```python
from build123d import *

# Parameters (mm, degrees)
SKETCH1_W           = 144
SKETCH1_H           = 71.25
BOSS_EXTRUDE1_DEPTH = 1
SKETCH2_W           = 13.75
SKETCH2_H           = 13.75
CUT_EXTRUDE1_DEPTH  = 81.33766629
SKETCH3_W           = 13.75
SKETCH3_H           = 13.75
CUT_EXTRUDE2_DEPTH  = 81.33766629
SKETCH4_W           = 7.5
SKETCH4_H           = 7.5
CUT_EXTRUDE6_DEPTH  = 81.33766629


with BuildPart() as part:
    # Sketch1 → Boss-Extrude1 (new body)
    with BuildSketch(Plane(origin=(0, 0, 0), x_dir=(1, 0, 0), z_dir=(0, 1, 0))):
        Rectangle(SKETCH1_W, SKETCH1_H)
    extrude(amount=BOSS_EXTRUDE1_DEPTH)

    # Sketch2 → Cut-Extrude1 (cut, through all)
    with BuildSketch(Plane(origin=(0, 1, 0), x_dir=(1, 0, 0), z_dir=(0, 1, 0))):
        with Locations((-36.375, 18.75)):
            Rectangle(SKETCH2_W, SKETCH2_H)
        with Locations((-55.125, 0)):
            Rectangle(SKETCH2_W, SKETCH2_H)
        with Locations((-36.375, -18.75)):
            Rectangle(SKETCH2_W, SKETCH2_H)
        with Locations((-17.625, 0)):
            Rectangle(SKETCH2_W, SKETCH2_H)
    cut_extrude1 = extrude(amount=-CUT_EXTRUDE1_DEPTH, mode=Mode.SUBTRACT)

    # Mirror1: Cut-Extrude1 across plane
    add(cut_extrude1.mirror(Plane(origin=(0, 0, 0), x_dir=(0, 0, 1), z_dir=(1, 0, 0))), mode=Mode.SUBTRACT)

    # Sketch3 → Cut-Extrude2 (cut, through all)
    with BuildSketch(Plane(origin=(0, 1, 0), x_dir=(1, 0, 0), z_dir=(0, 1, 0))):
        with Locations((0, 18.75)):
            Rectangle(SKETCH3_W, SKETCH3_H)
    extrude(amount=-CUT_EXTRUDE2_DEPTH, mode=Mode.SUBTRACT)

    # Sketch4 → Cut-Extrude6 (cut, through all)
    with BuildSketch(Plane(origin=(0, 1, 0), x_dir=(1, 0, 0), z_dir=(0, 1, 0))):
        with Locations((0, -16.379809472)):
            Rectangle(SKETCH4_W, SKETCH4_H)
        Polygon((0.05, -20.216412012), (-0.05, -20.216412012), (-1.375, -22.511379332), (-2.375, -24.24343014), (-3.75, -26.625), (-2.25, -26.625), (-0.25, -26.625), (0.25, -26.625), (2.25, -26.625), (3.75, -26.625), (2.375, -24.24343014), (1.375, -22.511379332), align=None)
        Polygon((5.339101615, -21.377404736), (1.375, -22.511379332), (2.375, -24.24343014), align=None)
        Polygon((-2.375, -24.24343014), (-1.375, -22.511379332), (-5.339101615, -21.377404736), align=None)
        Polygon((-0.25, -26.625), (-2.25, -26.625), (-1.25, -30.625), align=None)
        Polygon((1.25, -30.625), (2.25, -26.625), (0.25, -26.625), align=None)
        Polygon((-0.05, -20.216412012), (0, -20.129809472), (-0.05, -20.129809472), align=None)
        Polygon((0.05, -20.129809472), (0, -20.129809472), (0.05, -20.216412012), align=None)
        Polygon((0.05, -20.216412012), (0, -20.129809472), (-0.05, -20.216412012), align=None)
    extrude(amount=-CUT_EXTRUDE6_DEPTH, mode=Mode.SUBTRACT)


solid = part.part
```
Check sheet for the modelled part. Datum: model origin and axes. Units: mm. Coordinates: 2 decimals unless noted, no trailing zeros. Write each loop counter-clockwise with the first axis right and the second up, starting at its lowest first coordinate (ties: lowest second). Pieces come first, ordered by that corner, then holes. Notation, with made-up numbers: M 26.5,48 L 79.5,48 A23 ccw 79.5,71 Z; hole C -6.75,16 d8. An arc over 180 degrees is marked long. Write item = value, one per line. Start each with the question number.
1. Sectioned sample at A-A (x = -21). Record the cut outline in (y, z) (3 decimals).
2. Sectioned sample at D-D (y = 0.4). State how many separate pieces and enclosed holes the cut face has, then the cut area to 3 significant figures.
3. Sectioned sample at C-C (x = 33.5). Record the cut outline in (y, z) (3 decimals).
4. Mould release check, pull along X, two halves, no side actions. Record for faces 1 (the flat face through (3.836, 0.507, 22.83)), 2 (the flat face through (-3.88, 0.51, 22.79)), 3 (the flat face through (-1, 1, 0)): pulls with the +X half, pulls with the -X half, needs draft (parallel to the pull), parting line crosses it, or undercut.
5. Sectioned sample at B-B (z = 16). Record the cut outline in (x, y).
6. Thickness scan on probe 1 along X at (y, z) = (0.75, 18); probe 2 along Z at (x, y) = (40, 0.5) (3 decimals); probe 3 along X at (y, z) = (0.7, 6.5). Record the ranges inside material, lowest first.
The answers:
q1.outline = M 0,-35.625 L 1,-35.625 L 1,-6.875 L 0,-6.875 Z; M 0,6.875 L 1,6.875 L 1,35.625 L 0,35.625 Z
q2.separate_pieces = 1
q2.enclosed_holes = 10
q2.area = 8,460 mm²
q3.outline = M 0,-35.625 L 1,-35.625 L 1,-25.625 L 0,-25.625 Z; M 0,-11.875 L 1,-11.875 L 1,11.875 L 0,11.875 Z; M 0,25.625 L 1,25.625 L 1,35.625 L 0,35.625 Z
q4.face_1 = undercut
q4.face_2 = undercut
q4.face_3 = needs draft
q5.outline = M -72,0 L -43.25,0 L -43.25,1 L -72,1 Z; M -29.5,0 L -3.75,0 L -3.75,1 L -29.5,1 Z; M 3.75,0 L 29.5,0 L 29.5,1 L 3.75,1 Z; M 43.25,0 L 72,0 L 72,1 L 43.25,1 Z
q6.probe_1 = -72 to -43.25, -29.5 to -3.75, 3.75 to 29.5, 43.25 to 72
q6.probe_2 = -35.625 to -25.625, -11.875 to 11.875, 25.625 to 35.625
q6.probe_3 = -72 to -62, -48.25 to -24.5, -10.75 to 10.75, 24.5 to 48.25, 62 to 72
